Verification items for the finished model (mm, model axes). Face numbers are marked on the shaded views. A direction names the side the tool comes from. Round coordinates to 2 decimals unless told otherwise and drop trailing zeros. Write each loop counter-clockwise with the first axis right and the second up, starting at its lowest first coordinate (ties: lowest second). Pieces come first, ordered by that corner, then holes. Notation, with made-up numbers: M -28.75,-14.5 L 16.25,-14.5 A19 cw 16.25,10.5 Z; hole C 29,9.5 d8. An arc over 180 degrees is marked long. Answer in a Markdown table with one row per item. Add a question column.
1. Material ranges on probe 1 along X at (y, z) = (-6.5, -71.5); probe 2 along Z at (x, y) = (-31, -1.25); probe 3 along X at (y, z) = (-2.75, 24), recorded low to high.
2. Go/stop test with flat-tipped pins: pin 1 Ø5 at (x, y) = (-2.5, 7) entering from -Z; pin 2 Ø3 at (x, z) = (-8.5, -73) entering from +Y. Record where each tip stops, or that it passes through.
3. Set-up check for the marked faces 1 and 2: record each of +Z, -Z, +X, -X, +Y, -Y from which the full face is reachable in a straight line by a thin tool's end or side.
4. Sectioned sample at C-C on y = -2. Record the cut outline in (x, z), plus the area to 3 significant figures.
5. Sectioned sample at A-A on x = 31. Count the separate pieces of the cut face and the enclosed holes in it, plus the area to 3 significant figures.
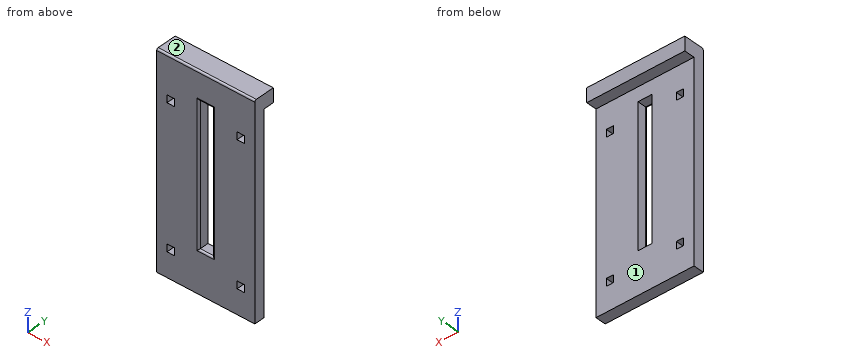
```python
from build123d import *

# Parameters (mm, degrees)
F0_W     = 88.9
F0_H     = 190.5
F0_W_2   = 6.731
F0_H_2   = 6.731
F0_W_3   = 12.7
F0_H_3   = 127
F1_DEPTH = 9.525
F2_R     = 1.5875
F3_W     = 9.525
F3_H     = 12.7
F4_DEPTH = 44.45


with BuildPart() as f1:
    # F0 (on Front) → F1 (new body)
    with BuildSketch(Plane.XZ):
        Rectangle(F0_W, F0_H)
        with Locations((-31.75, -69.85)):
            Rectangle(F0_W_2, F0_H_2, mode=Mode.SUBTRACT)
        with Locations((31.75, -69.85)):
            Rectangle(F0_W_2, F0_H_2, mode=Mode.SUBTRACT)
        with Locations((-31.75, 57.15)):
            Rectangle(F0_W_2, F0_H_2, mode=Mode.SUBTRACT)
        with Locations((0, 6.35)):
            Rectangle(F0_W_3, F0_H_3, mode=Mode.SUBTRACT)
        with Locations((31.75, 57.15)):
            Rectangle(F0_W_2, F0_H_2, mode=Mode.SUBTRACT)
    extrude(amount=F1_DEPTH)

    # F2
    f2_edges = [f1.edges().sort_by_distance(p)[0] for p in [
        (0, -9.525, 95.25),
        (-6.35, -9.525, 6.35),
        (6.35, -9.525, 6.35),
        (0, -9.525, 69.85),
        (0, -9.525, -57.15),
    ]]
    fillet(f2_edges, radius=F2_R)

    # F3 (on Right) → F4 (join, symmetric)
    with BuildSketch(Plane.YZ):
        with Locations((4.7625, 88.9)):
            Rectangle(F3_W, F3_H)
    extrude(amount=F4_DEPTH, both=True)


solid = f1.part
```
Geometry check:
| question | item | result |
|---|---|---|
| 1 | probe 1 | x = -44.45 to -35.12, -28.38 to 28.38, 35.12 to 44.45 |
| 1 | probe 2 | z = -95.25 to -73.22, -66.48 to 53.78, 60.52 to 95.25 |
| 1 | probe 3 | x = -44.45 to -6.35, 6.35 to 44.45 |
| 2 | pin 1 | stops at z = 82.55 |
| 2 | pin 2 | stops at y = 0 |
| 3 | face 1 | -Z, +X, -X, +Y |
| 3 | face 2 | +Z, +X, -X, +Y, -Y |
| 4 | outline | M -44.45,-95.25 L 44.45,-95.25 L 44.45,95.25 L -44.45,95.25 Z; hole M -35.12,-73.22 L -28.38,-73.22 L -28.38,-66.48 L -35.12,-66.48 Z; hole M -35.12,53.78 L -28.38,53.78 L -28.38,60.52 L -35.12,60.52 Z; hole M -6.35,-57.15 L 6.35,-57.15 L 6.35,69.85 L -6.35,69.85 Z; hole M 28.38,-73.22 L 35.12,-73.22 L 35.12,-66.48 L 28.38,-66.48 Z; hole M 28.38,53.78 L 35.12,53.78 L 35.12,60.52 L 28.38,60.52 Z |
| 4 | area | 15,100 mm2 |
| 5 | separate pieces | 3 |
| 5 | enclosed holes | 0 |
| 5 | area | 1,810 mm2 |
